```python
from build123d import *

# Parameters (mm, degrees)
F1_DEPTH = 6.42
F2_R     = 6.345
F3_DEPTH = 34
F4_R     = 6.345
F5_DEPTH = 18.2
F7_DEPTH = 18.2


with BuildPart() as f1:
    # F0 (on Top) → F1 (new body)
    with BuildSketch(Plane.XY):
        with BuildLine():
            Line((5, 15.1), (-5, 15.1))
            ThreePointArc((-5, 15.1), (-20.1, 0), (-5, -15.1))
            Line((-5, -15.1), (5, -15.1))
            ThreePointArc((5, -15.1), (20.1, 0), (5, 15.1))
        make_face()
    extrude(amount=F1_DEPTH)

    # F2 (on face) → F3 (join)
    with BuildSketch(Plane(origin=(0, 0, 0), x_dir=(1, 0, 0), z_dir=(0, 0, -1))):
        Circle(F2_R)
    extrude(amount=F3_DEPTH)

    # F4 (on face) → F5 (join)
    with BuildSketch(Plane.XY.offset(6.42)):
        Circle(F4_R)
    extrude(amount=F5_DEPTH)

    # F6 (on face) → F7 (cut)
    with BuildSketch(Plane.XY.offset(24.62)):
        with BuildLine():
            ThreePointArc((-3.821623, -5.065), (-2.015143, -6.016496), (0, -6.345))
            Line((0, -6.345), (0, -5.065))
            Line((0, -5.065), (-3.821623, -5.065))
        make_face()
        with BuildLine():
            Line((0, -5.065), (0, -6.345))
            ThreePointArc((0, -6.345), (2.015143, -6.016496), (3.821623, -5.065))
            Line((3.821623, -5.065), (0, -5.065))
        make_face()
    extrude(amount=-F7_DEPTH, mode=Mode.SUBTRACT)


solid = f1.part
```
For this review, take the finished solid that the model builds, in its own axes (mm). A direction names the side the tool comes from. Coordinates: 2 decimals unless noted, no trailing zeros. Loops run counter-clockwise (first coordinate to the right, second up) from the corner with the lowest first, then second, coordinate; pieces in that order, holes last. Notation, with made-up numbers: (12, 75) - (38, 75) arc R23 ccw to (38, 99) - close; hole circle Ø9 at (-20, 3). An arc over 180 degrees is marked (long way). Use one line per item in the form item = value. Start each with the question number.
1) For pin 1 (8.5 mm diameter, centred on x = -1, z = 16.5, fed in from -Y) (3 decimals); pin 2 (12 mm diameter, centred on x = -6.5, z = -23.5, fed in from +Y); pin 3 (5 mm diameter, centred on x = -11.5, y = -3, fed in from -Z), all flat-tipped, find the tip position at first contact; note any pin that passes through.
2) To check wall thickness, follow probe 1 along Z at (x, y) = (-10, -2.5); probe 2 along X at (y, z) = (-0.5, 5.5); probe 3 along Y at (x, z) = (-3, -14.5). State the ranges of each line that lie inside material, in increasing order. Write a range as from..to.
3) Take a section at D-D (y = -8). State the section outline as (x, z) points.
4) For faces 1 (the face through (0, 0, -34)), 2 (the face through (0, 7, 6.42)), 3 (the face through (-0.83, -6.29, -16.76)), list the 3-axis set-ups (+Z, -Z, +X, -X, +Y, -Y) from which the entire face can be reached by the end or side of a thin tool; tool diameter is ignored.
5) Take a section at A-A (x = 0). State the section outline as (y, z) points (3 decimals).
6) Draft analysis for pull direction Y (two halves, no side actions). For faces 4 (the face through (0, 7, 0)), 5 (the face through (-20.096, 0.332, 3.165)), 6 (the face through (0, -5.065, 16)), state which applies: released by +Y, released by -Y, zero draft, split by the parting line, or undercut.
7) Take a section at B-B (y = 0). State the section outline as (x, z) points (3 decimals), plus the area to 4 significant figures.
8) Take a section at C-C (z = -22). State the section outline as (x, y) points (3 decimals).
From the geometry:
q1.pin_1 = -5.065
q1.pin_2 = 6.33
q1.pin_3 = 0
q2.probe_1 = 0..6.42
q2.probe_2 = -20.09..20.09
q2.probe_3 = -5.59..5.59
q3.outline = (-17.81, 0) - (17.81, 0) - (17.81, 6.42) - (-17.81, 6.42) - close
q4.face_1 = -Z, +X, -X, +Y, -Y
q4.face_2 = +Z
q4.face_3 = -Z
q5.outline = (-15.1, 0) - (-6.345, 0) - (-6.345, -34) - (6.345, -34) - (6.345, 0) - (15.1, 0) - (15.1, 6.42) - (6.345, 6.42) - (6.345, 24.62) - (-5.065, 24.62) - (-5.065, 6.42) - (-15.1, 6.42) - close
q6.face_4 = zero draft
q6.face_5 = split by the parting line
q6.face_6 = released by -Y
q7.outline = (-20.1, 0) - (-6.345, 0) - (-6.345, -34) - (6.345, -34) - (6.345, 0) - (20.1, 0) - (20.1, 6.42) - (6.345, 6.42) - (6.345, 24.62) - (-6.345, 24.62) - (-6.345, 6.42) - (-20.1, 6.42) - close
q7.area = 920.5 mm2
q8.outline = circle Ø12.69 at (0, 0)
